```python
from build123d import *

# Parameters (mm, degrees)
EXTRUDE_1_DEPTH                = 20
SKETCH_2_4_R                   = 50
EXTRUDE_2_DEPTH                = 40
EXTRUDE_3_DEPTH                = 10
FILLET_1_R                     = 10
HOLE_WIZARD_M1_6_1_D           = 25
HOLE_WIZARD_M1_6_1_CBORE_D     = 50
HOLE_WIZARD_M1_6_1_CBORE_DEPTH = 15


with BuildPart() as part:
    # Sketch 2 → Extrude 1 (new body)
    with BuildSketch(Plane(origin=(0, 0, 0), x_dir=(1, 0, 0), z_dir=(0, 1, 0))):
        with BuildLine():
            Line((180, 50), (0, 50))
            ThreePointArc((0, 50), (35.355339059, 35.355339059), (50, 0))
            ThreePointArc((50, 0), (49.74680765, -5.0254481), (48.989794856, -10))
            Line((48.989794856, -10), (180, -10))
            Line((180, -10), (180, 50))
        make_face()
        with BuildLine():
            ThreePointArc((60, 0), (56.050341538, 21.409325386), (44.72135955, 40))
            Line((44.72135955, 40), (170, 40))
            Line((170, 40), (170, 0))
            Line((170, 0), (60, 0))
        make_face(mode=Mode.SUBTRACT)
    extrude(amount=EXTRUDE_1_DEPTH)

    # Sketch 2_4 → Extrude 2 (add)
    with BuildSketch(Plane(origin=(0, 0, 0), x_dir=(1, 0, 0), z_dir=(0, 1, 0))):
        Circle(SKETCH_2_4_R)
    extrude(amount=EXTRUDE_2_DEPTH)

    # Sketch 2_5 → Extrude 3 (add)
    with BuildSketch(Plane(origin=(0, 0, 0), x_dir=(1, 0, 0), z_dir=(0, 1, 0))):
        with BuildLine():
            Line((44.72135955, 40), (170, 40))
            Line((170, 40), (170, 0))
            Line((170, 0), (60, 0))
            ThreePointArc((60, 0), (56.050341538, 21.409325386), (44.72135955, 40))
        make_face()
    extrude(amount=EXTRUDE_3_DEPTH)

    # Fillet 1
    fillet_1_edges = [part.edges().sort_by_distance(p)[0] for p in [
        (170, 15, 0),
        (170, 15, -40),
        (180, 10, -50),
        (180, 10, 10),
    ]]
    fillet(fillet_1_edges, radius=FILLET_1_R)

    # Hole Wizard M1.6 _ _ _ _1 (through all)
    with Locations(Plane(origin=(0, 40, 0), x_dir=(1, 0, 0), z_dir=(0, 1, 0))):
        with Locations((0, 0)):
            CounterBoreHole(HOLE_WIZARD_M1_6_1_D / 2, HOLE_WIZARD_M1_6_1_CBORE_D / 2, HOLE_WIZARD_M1_6_1_CBORE_DEPTH)


solid = part.part
```
Read the model definition and answer for the solid it produces. Units are mm, in the model's axes. A direction names the side the tool comes from. Coordinates: 2 decimals unless noted, no trailing zeros. Loops run counter-clockwise (first coordinate to the right, second up) from the corner with the lowest first, then second, coordinate; pieces in that order, holes last.
(1) The part is cut by section B-B (z = -34.5). Determine the outline of the cut face in (x, y).
Solution:
outline: (-36.19, 0) - (180, 0) - (180, 20) - (168.93, 20) - (168.93, 10) - (49.09, 10) - (49.09, 20) - (36.19, 20) - (36.19, 40) - (-36.19, 40) - close
(2) A tool of negligible diameter and unlimited length cuts with its end or side. For faces 1 (the face through (-5.9, 25, -11.5)), 2 (the face through (109, 10, 10)), 3 (the face through (67, 0, -12)), from which of +Z, -Z, +X, -X, +Y, -Y can it reach the whole face along a straight path? Write none if from no direction.
Solution:
face 1: +Y
face 2: +Z, +X, +Y, -Y
face 3: +Z, -Z, +X, -X, -Y
(3) The mould has two halves that part along X. Classify faces 4 (the face through (86, 10, -50)), 5 (the face through (56.16, 14.93, -21.12)), 6 (the face through (180, 10, -20)): released by +X, released by -X, zero draft, split by the parting line, or undercut.
Solution:
face 4: zero draft
face 5: undercut
face 6: released by +X
(4) The part is cut by section D-D (z = -15.5). Determine the outline of the cut face in (x, y), and give its area (3 significant figures).
Solution:
outline: (-47.54, 0) - (180, 0) - (180, 20) - (170, 20) - (170, 10) - (57.96, 10) - (57.96, 20) - (47.54, 20) - (47.54, 40) - (19.62, 40) - (19.62, 25) - (-19.62, 25) - (-19.62, 40) - (-47.54, 40) - close
area: 4,740 mm2
(5) Consider line 1 along Z through (x, y) = (0, 36); line 2 along Z through (x, y) = (156, 15.5); line 3 along Y through (x, z) = (70, 4.5). Determine where each line is inside the solid, lowest interval first.
Solution:
line 1: z = -50 to -25, 25 to 50
line 2: z = -50 to -40, 0 to 10
line 3: y = 0 to 20
(6) Flat-ended cylindrical pins translate along their axes: pin 1 Ø3 at (y, z) = (31, -38) entering from +X; pin 2 Ø6 at (x, z) = (61.5, 5) entering from +Y; pin 3 Ø3 at (y, z) = (15, -21) entering from -X. Find the tip coordinate at first contact, or state that the pin passes through.
Solution:
pin 1: stops at x = 34.17
pin 2: stops at y = 20
pin 3: stops at x = -46.04
(7) The part is cut by section C-C (y = 34). Determine the outline of the cut face in (x, z).
Solution:
outline: circle Ø100 at (0, 0); hole circle Ø50 at (0, 0)
(8) The part is cut by section A-A (x = 93). Determine the outline of the cut face in (y, z).
Solution:
outline: (0, -50) - (20, -50) - (20, -40) - (10, -40) - (10, 0) - (20, 0) - (20, 10) - (0, 10) - close
